Source: CAD feature listing. Evaluate the final solid. Frame: model axes, mm. A direction names the side the tool comes from. Coordinates: 2 decimals unless noted, no trailing zeros. Order: outer loops, then holes, each group sorted by start corner. A loop starts at its lowest first (then second) coordinate and runs counter-clockwise, first axis right, second up.
```python
from build123d import *

# Parameters (mm, degrees)
F0_W        = 43.0329442024
F0_H        = 82.2901595384
F1_DEPTH    = 135.636
F2_T1_DEPTH = 212.9316553271
F3_W        = 19.7290945798
F3_H        = 38.1281389855
F3_R        = 12.2243381544
F3_R_2      = 14.5784118216
F3_R_3      = 9.3761022788
F4_DEPTH    = 9.652


# Not quite as in the source:
# - a fillet or chamfer that OpenCascade refuses, or shapes differently, is made with other operations: its cross-section is extruded or revolved along the edge and cut away or added


with BuildPart() as f1:
    # F0 (on Top) → F1 (new body)
    with BuildSketch(Plane.XY):
        with Locations((-110.2483123541, 24.9322196469)):
            Rectangle(F0_W, F0_H)
    extrude(amount=F1_DEPTH)

    # F2: chamfer of 25.4 on 2 edges, made by hand

    # F2_s2 → F2_t1 (cut)
    with BuildSketch(Plane.XZ.offset(-131.3980473104)):
        Polygon((-131.7647844553, 110.236), (-106.3647844553, 135.636), (-131.7647844553, 135.636), align=None)
        Polygon((-88.7318402529, 110.236), (-114.1318402529, 135.636), (-88.7318402529, 135.636), align=None)
    extrude(amount=F2_T1_DEPTH, mode=Mode.SUBTRACT)

    # F3 (on face) → F4 (cut)
    with BuildSketch(Plane(origin=(-131.7647844553, 0, 0), x_dir=(0, -1, 0), z_dir=(-1, 0, 0))):
        with Locations((-38.9040028676, 23.8969207276)):
            Rectangle(F3_W, F3_H)
        with Locations((-51.650326699, 87.2960314155)):
            Circle(F3_R)
        with Locations((-8.8670095429, 87.961062789)):
            Circle(F3_R_2)
        with Locations((-3.9901542477, 25.8919987828)):
            Circle(F3_R_3)
    extrude(amount=-F4_DEPTH, mode=Mode.SUBTRACT)


solid = f1.part
```
1. Draft query along Y for faces 3 (the face through (-122.113, 39, 24)), 4 (the face through (-111, -16.213, 65)), 5 (the face through (-127.01, 12.03, 73.73)), 6 (the face through (-111, 26, 0)). Return one class per face: released by +Y, released by -Y, zero draft, split by the parting line, or undercut.
Findings:
face 3: undercut
face 4: released by -Y
face 5: undercut
face 6: zero draft
2. Access query for faces 1 (the face through (-122.113, 9, 88)), 2 (the face through (-88.732, 24, 54)). Directions: +Z, -Z, +X, -X, +Y, -Y. A direction counts if a zero-diameter tool reaches every point of the face in a straight line with its end or side. Return the directions, or none.
Findings:
face 1: -X
face 2: +Z, -Z, +X, +Y, -Y
3. Pin query (flat end, axial travel): P1, Ø10, axis at x = -124.5, y = 41, coming from the -Z side; P2, Ø6, axis at y = 40.5, z = 21.5, coming from the -X side; P3, Ø7.5, axis at x = -127, y = 43, coming from the +Z side. Return the tip coordinate at first contact, or that it passes through.
Findings:
P1: stops at z = 0
P2: stops at x = -122.11
P3: stops at z = 118.75
4. Section query D-D on x = -101. Return loops of the section in (y, z).
Findings:
outline: (-16.21, 0) - (66.08, 0) - (66.08, 122.5) - (-16.21, 122.5) - close
5. Section query C-C on x = -126.5. Return loops of the section in (y, z).
Findings:
outline: (-16.21, 0) - (66.08, 0) - (66.08, 115.5) - (-16.21, 115.5) - close; hole circle Ø29.16 at (8.87, 87.96); hole circle Ø18.75 at (3.99, 25.89); hole (29.04, 4.83) - (48.77, 4.83) - (48.77, 42.96) - (29.04, 42.96) - close; hole circle Ø24.45 at (51.65, 87.3)
6. Ray query, line 1 (X direction, y = 18.5, z = 83.5); line 2 (Z direction, x = -127, y = 61.5); line 3 (X direction, y = 54, z = 116). Return the intervals inside material, ascending.
Findings:
line 1: x = -122.11 to -88.73
line 2: z = 0 to 80.06, 94.54 to 115
line 3: x = -126 to -94.5
7. Section query B-B on y = 37. Return loops of the section in (x, z).
Findings:
outline: (-131.76, 0) - (-88.73, 0) - (-88.73, 110.24) - (-110.25, 131.75) - (-131.76, 110.24) - (-131.76, 42.96) - (-122.11, 42.96) - (-122.11, 4.83) - (-131.76, 4.83) - close
8. Section query A-A on z = 14. Return loops of the section in (x, y), plus the area to 3 significant figures.
Findings:
outline: (-131.76, -16.21) - (-88.73, -16.21) - (-88.73, 66.08) - (-131.76, 66.08) - (-131.76, 48.77) - (-122.11, 48.77) - (-122.11, 29.04) - (-131.76, 29.04) - close
area: 3,350 mm2
